```python
from build123d import *

# Parameters (mm, degrees)
BOSS_EXTRUDE1_DEPTH  = 250
M4_CLEARANCE_HOLE1_D = 4.5
LPATTERN1_COUNT      = 5
LPATTERN1_PITCH      = 57.5


with BuildPart() as part:
    # Sketch1 → Boss-Extrude1 (new body)
    with BuildSketch(Plane(origin=(0, 0, 0), x_dir=(0, 0, -1), z_dir=(1, 0, 0))):
        Polygon((-5, 23), (0, 28), (0, 0), (-5, 0), align=None)
    extrude(amount=BOSS_EXTRUDE1_DEPTH)

    # M4 Clearance Hole1 (through all)
    with Locations(Plane.XY.offset(5)):
        with Locations((10, 9)):
            m4_clearance_hole1 = Hole(M4_CLEARANCE_HOLE1_D / 2)

    # LPattern1: M4 Clearance Hole1 ×5
    with Locations(*[(i * LPATTERN1_PITCH, 0, 0) for i in range(1, LPATTERN1_COUNT)]):
        add(m4_clearance_hole1, mode=Mode.SUBTRACT)


solid = part.part
```
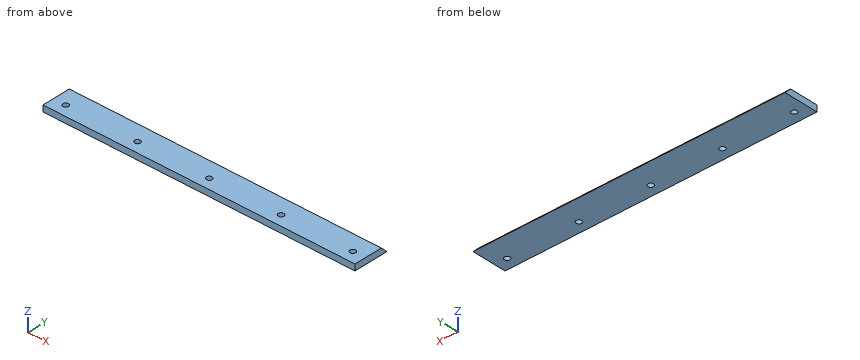
CAD build for the part. Positions are in the model's coordinates, mm. Round coordinates to 2 decimals unless told otherwise and drop trailing zeros. Write each loop counter-clockwise with the first axis right and the second up, starting at its lowest first coordinate (ties: lowest second). Pieces come first, ordered by that corner, then holes. Notation, with made-up numbers: (19.25, 44.25) - (37.25, 44.25) arc R15 ccw to (37.25, 52.25) - close; hole circle Ø2 at (49, 27). An arc over 180 degrees is marked (long way). Return JSON: item names as keys, results as strings. Group by question number.
Item 1: Band-saw the part on A-A on z = 2.1. List the corners of the cut face in (x, y), plus the area to 3 significant figures.
Item 2: Probe probe 1 along X at (y, z) = (8.75, 2.7); probe 2 along Y at (x, z) = (182.5, 1.55); probe 3 along Y at (x, z) = (125, 1.65). List the from-to ranges inside material, lowest first.
Item 3: Band-saw the part on B-B on x = 240. List the corners of the cut face in (y, z), plus the area to 3 significant figures.
Item 4: Band-saw the part on D-D on x = 109.5. List the corners of the cut face in (y, z).
Item 5: Band-saw the part on C-C on y = 9. List the corners of the cut face in (x, z), plus the area to 3 significant figures.
Resolved:
{
 "1": {"outline": "(0, 0) - (250, 0) - (250, 25.9) - (0, 25.9) - close; hole circle Ø4.5 at (10, 9); hole circle Ø4.5 at (67.5, 9); hole circle Ø4.5 at (125, 9); hole circle Ø4.5 at (182.5, 9); hole circle Ø4.5 at (240, 9)", "area": "6,400 mm²"},
 "2": {"probe 1": "x = 0 to 7.76, 12.24 to 65.26, 69.74 to 122.76, 127.24 to 180.26, 184.74 to 237.76, 242.24 to 250", "probe 2": "y = 0 to 6.75, 11.25 to 26.45", "probe 3": "y = 0 to 6.75, 11.25 to 26.35"},
 "3": {"outline": "(0, 0) - (6.75, 0) - (6.75, 5) - (0, 5) - close; (11.25, 0) - (28, 0) - (23, 5) - (11.25, 5) - close", "area": "105 mm²"},
 "4": {"outline": "(0, 0) - (28, 0) - (23, 5) - (0, 5) - close"},
 "5": {"outline": "(0, 0) - (7.75, 0) - (7.75, 5) - (0, 5) - close; (12.25, 0) - (65.25, 0) - (65.25, 5) - (12.25, 5) - close; (69.75, 0) - (122.75, 0) - (122.75, 5) - (69.75, 5) - close; (127.25, 0) - (180.25, 0) - (180.25, 5) - (127.25, 5) - close; (184.75, 0) - (237.75, 0) - (237.75, 5) - (184.75, 5) - close; (242.25, 0) - (250, 0) - (250, 5) - (242.25, 5) - close", "area": "1,140 mm²"}
}
